from build123d import *

# Parameters (mm, degrees)
SKETCH1_R           = 4
BOSS_EXTRUDE1_DEPTH = 5
BOSS_EXTRUDE2_DEPTH = 7
SKETCH3_R           = 4
BOSS_EXTRUDE3_DEPTH = 5
BOSS_EXTRUDE4_START = -17
BOSS_EXTRUDE4_DEPTH = 17
SKETCH5_W           = 20
SKETCH5_H           = 33
BOSS_EXTRUDE5_DEPTH = 5


with BuildPart() as part:
    # Sketch1 → Boss-Extrude1 (new body)
    with BuildSketch(Plane.XY):
        with BuildLine():
            Line((-50, 0), (-10, 0))
            ThreePointArc((-10, 0), (0, 10), (10, 0))
            Line((10, 0), (50, 0))
            ThreePointArc((50, 0), (0, -50), (-50, 0))
        make_face()
        Circle(SKETCH1_R, mode=Mode.SUBTRACT)
    extrude(amount=BOSS_EXTRUDE1_DEPTH)

    # Sketch2 → Boss-Extrude2 (add)
    with BuildSketch(Plane.XY.offset(5)):
        with BuildLine():
            Line((-50, 0), (-40, 0))
            ThreePointArc((-40, 0), (0, -40), (40, 0))
            Line((40, 0), (50, 0))
            ThreePointArc((50, 0), (0, -50), (-50, 0))
        make_face()
    extrude(amount=BOSS_EXTRUDE2_DEPTH)

    # Sketch3 → Boss-Extrude3 (add)
    with BuildSketch(Plane.XY.offset(12)):
        with BuildLine():
            Line((-50, 0), (-10, 0))
            ThreePointArc((-10, 0), (0, 10), (10, 0))
            Line((10, 0), (50, 0))
            ThreePointArc((50, 0), (0, -50), (-50, 0))
        make_face()
        Circle(SKETCH3_R, mode=Mode.SUBTRACT)
    extrude(amount=BOSS_EXTRUDE3_DEPTH)

    # Sketch4 → Boss-Extrude4 (add)
    with BuildSketch(Plane.XY.offset(17).offset(BOSS_EXTRUDE4_START)):
        with BuildLine():
            Line((-10, -88.989794856), (10, -88.989794856))
            Line((10, -88.989794856), (10, -48.989794856))
            ThreePointArc((10, -48.989794856), (0, -50), (-10, -48.989794856))
            Line((-10, -48.989794856), (-10, -88.989794856))
        make_face()
    extrude(amount=BOSS_EXTRUDE4_DEPTH)

    # Sketch5 → Boss-Extrude5 (add)
    with BuildSketch(Plane.XZ.offset(88.989794856)):
        with Locations((0, 0.5)):
            Rectangle(SKETCH5_W, SKETCH5_H)
    extrude(amount=BOSS_EXTRUDE5_DEPTH)


solid = part.part
Could you check a few things on this model? Use its own coordinates, in mm. A direction names the side the tool comes from. Give positions to 0.01 mm unless a question says otherwise; leave off trailing zeros. Order: outer loops, then holes, each group sorted by start corner. A loop starts at its lowest first (then second) coordinate and runs counter-clockwise, first axis right, second up. Notation, with made-up numbers: (9.5, 44) -> (30.5, 44) arc R31 cw to (30.5, 72) -> close; hole circle Ø4 at (52.5, -4.75). An arc over 180 degrees is marked (long way). Answer in a Markdown table with one row per item. Add a question column.
Item 1: Imagine slicing it at D-D (y = -61). List the corners of the cut face in (x, z) for me.
Item 2: I'm going to push flat-ended pins straight in: P1, Ø2, axis at x = 20, z = 0.5, coming from the -Y side; P2, Ø2, axis at x = 16, z = 9.5, coming from the -Y side; P3, Ø10, axis at x = -38.5, z = -1.5, coming from the +Y side. Where does each tip first touch, or does it pass through?
Item 3: Imagine slicing it at C-C (x = 15.5). List the corners of the cut face in (y, z) for me, and give its area (3 significant figures).
Item 4: We'd pull the mould along X, two halves only. Please class faces 1 (the cylindrical face through (-0.867, -3.905, 14.465)), 2 (the cylindrical face through (0, 10, 14)), 3 (the cylindrical face through (39.03, -31.25, 8.38)): pulls with the +X half, pulls with the -X half, needs draft (parallel to the pull), parting line crosses it, or undercut.
Item 5: Please list where these lines run through material, in increasing order: probe 1 along Y at (x, z) = (0, 2.7); probe 2 along Z at (x, y) = (27.5, -5); probe 3 along Z at (x, y) = (3, -41).
Item 6: Imagine slicing it at A-A (x = 0). List the corners of the cut face in (y, z) for me, and give its area (3 significant figures).
Item 7: For faces 4 (the flat face through (-30.3, 0, 4.6)), 5 (the flat face through (-10, -71, 8)), 6 (the flat face through (0, -88.99, -8)), 7 (the flat face through (10, -71, 8)), which set-ups out of +Z, -Z, +X, -X, +Y, -Y let a thin tool reach every point of the face, with its end or its side?
Item 8: Imagine slicing it at B-B (y = -36). List the corners of the cut face in (x, z) for me.
Result:
| question | item | result |
|---|---|---|
| 1 | outline | (-10, 0) -> (10, 0) -> (10, 17) -> (-10, 17) -> close |
| 2 | P1 | y = -46.25 |
| 2 | P2 | y = -47.7 |
| 2 | P3 | y = 0 |
| 3 | outline | (-47.54, 0) -> (0, 0) -> (0, 5) -> (-36.87, 5) -> (-36.87, 12) -> (0, 12) -> (0, 17) -> (-47.54, 17) -> close |
| 3 | area | 550 mm2 |
| 4 | face 1 | undercut |
| 4 | face 2 | parting line crosses it |
| 4 | face 3 | pulls with the +X half |
| 5 | probe 1 | -93.99 to -4, 4 to 10 |
| 5 | probe 2 | 0 to 5, 12 to 17 |
| 5 | probe 3 | 0 to 17 |
| 6 | outline | (-93.99, -16) -> (-88.99, -16) -> (-88.99, 0) -> (-4, 0) -> (-4, 5) -> (-40, 5) -> (-40, 12) -> (-4, 12) -> (-4, 17) -> (-93.99, 17) -> close; (4, 0) -> (10, 0) -> (10, 5) -> (4, 5) -> close; (4, 12) -> (10, 12) -> (10, 17) -> (4, 17) -> close |
| 6 | area | 1,420 mm2 |
| 7 | face 4 | +Z, -Z, -X, +Y |
| 7 | face 5 | +Z, -Z, -X, -Y |
| 7 | face 6 | -Z, +X, -X, +Y |
| 7 | face 7 | +Z, -Z, +X, -Y |
| 8 | outline | (-34.7, 0) -> (34.7, 0) -> (34.7, 17) -> (-34.7, 17) -> close; hole (-17.44, 5) -> (17.44, 5) -> (17.44, 12) -> (-17.44, 12) -> close |
